Can you work these out from the model? Positions are in its coordinate system, mm. Coordinates: 2 decimals unless noted, no trailing zeros. Order: outer loops, then holes, each group sorted by start corner. A loop starts at its lowest first (then second) coordinate and runs counter-clockwise, first axis right, second up. Notation, with made-up numbers: M 58.5,13 L 111.5,13 A10 ccw 111.5,26 Z; hole C -33.5,45 d7. An arc over 180 degrees is marked long. Answer as a JSON object with one key per item and string values.
from build123d import *

# Parameters (mm, degrees)
SKETCH_1_W                  = 25
SKETCH_1_H                  = 25
EXTRUDE_1_DEPTH             = 4.5
SKETCH_2_R                  = 1.7
CUT_EXTRUDE_1_DEPTH         = 19.241436347
PATTERN_LINEAR_1_COUNT      = 2
PATTERN_LINEAR_1_PITCH      = 15
PATTERN_LINEAR_1_COUNT_DIR2 = 2
PATTERN_LINEAR_1_PITCH_DIR2 = 15
CHAMFER_1_SIZE              = 0.2


with BuildPart() as part:
    # 草圖1 → 填料-伸長1 (new body)
    with BuildSketch(Plane.XY):
        Rectangle(SKETCH_1_W, SKETCH_1_H)
    extrude(amount=EXTRUDE_1_DEPTH)

    # 草圖2 → 除料-伸長1 (cut, through all)
    with BuildSketch(Plane(origin=(0, 0, 0), x_dir=(-1, 0, 0), z_dir=(0, 0, -1))):
        with Locations((-7.5, 7.5)):
            Circle(SKETCH_2_R)
    cut_extrude_1 = extrude(amount=-CUT_EXTRUDE_1_DEPTH, mode=Mode.SUBTRACT)

    # 直線複製排列1: Cut-Extrude 1 2 × 2
    with Locations(*[(-i * PATTERN_LINEAR_1_PITCH, -j * PATTERN_LINEAR_1_PITCH_DIR2, 0) for i in range(PATTERN_LINEAR_1_COUNT) for j in range(PATTERN_LINEAR_1_COUNT_DIR2) if (i, j) != (0, 0)]):
        add(cut_extrude_1, mode=Mode.SUBTRACT)

    # 導角1
    chamfer_1_edges = [part.edges().sort_by_distance(p)[0] for p in [
        (9.2, 7.5, 0),
        (-5.8, 7.5, 0),
        (9.2, -7.5, 0),
        (-5.8, -7.5, 0),
        (0, 12.5, 0),
        (0, -12.5, 0),
    ]]
    chamfer(chamfer_1_edges, length=CHAMFER_1_SIZE)


solid = part.part
Item 1: I want a section at C-C, the plane z = 0.85. Write out the boundary of the cut face in (x, y).
Answers follow:
{"outline": "M -12.5,-12.5 L 12.5,-12.5 L 12.5,12.5 L -12.5,12.5 Z; hole C -7.5,-7.5 d3.4; hole C -7.5,7.5 d3.4; hole C 7.5,-7.5 d3.4; hole C 7.5,7.5 d3.4"}
Item 2: I want a section at B-B, the plane x = 7.5. Write out the boundary of the cut face in (y, z), plus the area to 3 significant figures.
Answers follow:
{"outline": "M -12.5,0.2 L -12.3,0 L -9.4,0 L -9.2,0.2 L -9.2,4.5 L -12.5,4.5 Z; M -5.8,0.2 L -5.6,0 L 5.6,0 L 5.8,0.2 L 5.8,4.5 L -5.8,4.5 Z; M 9.2,0.2 L 9.4,0 L 12.3,0 L 12.5,0.2 L 12.5,4.5 L 9.2,4.5 Z", "area": "81.8 mm^2"}
Item 3: Please list where these lines run through material, in increasing order: line 1 (Y direction, x = -7.5, z = 1.75); line 2 (X direction, y = -9, z = 1.15); line 3 (Y direction, x = 8, z = 0.9).
Answers follow:
{"line 1": "y = -12.5 to -9.2, -5.8 to 5.8, 9.2 to 12.5", "line 2": "x = -12.5 to -8.3, -6.7 to 6.7, 8.3 to 12.5", "line 3": "y = -12.5 to -9.12, -5.88 to 5.88, 9.12 to 12.5"}
Item 4: If we mould it in two halves opening along Y, with no side actions, what happens to faces 1 (the flat face through (0, -12.5, 2)), 2 (the flat face through (0, 0, 4.5)), 3 (the cylindrical face through (-7.13, -9.16, 2.32))? For each: pulls with the +Y half, pulls with the -Y half, needs draft (parallel to the pull), parting line crosses it, or undercut.
Answers follow:
{"face 1": "pulls with the -Y half", "face 2": "needs draft", "face 3": "undercut"}
Item 5: I want a section at A-A, the plane y = -7.5. Write out the boundary of the cut face in (x, z).
Answers follow:
{"outline": "M -12.5,0 L -9.4,0 L -9.2,0.2 L -9.2,4.5 L -12.5,4.5 Z; M -5.8,0.2 L -5.6,0 L 5.6,0 L 5.8,0.2 L 5.8,4.5 L -5.8,4.5 Z; M 9.2,0.2 L 9.4,0 L 12.5,0 L 12.5,4.5 L 9.2,4.5 Z"}
Item 6: I want a section at D-D, the plane y = 8. Give the number of separate pieces and of enclosed holes in the cut face, plus the area to 3 significant figures.
Answers follow:
{"separate pieces": "3", "enclosed holes": "0", "area": "83.2 mm^2"}
